```python
from build123d import *

# Parameters (mm, degrees)
F4_DEPTH  = 28.2
F5_R      = 3.9039510248
F6_DEPTH  = 25.8
F7_R      = 5.1903964383
F8_DEPTH  = 37
F10_DEPTH = 2.3
F11_R     = 18.8791722518
F12_DEPTH = 1.5
F13_W     = 2.7272701263
F13_H     = 4.5454557985
F15_R     = 5.8210220824
F16_DEPTH = 19.1
F17_R     = 3.5573808127
F18_DEPTH = 30


with BuildPart() as f1:
    # F0 (on Front) → F1 (revolve)
    with BuildSketch(Plane.XZ):
        with BuildLine():
            Line((-15.875, -15.875), (0, -15.875))
            Line((0, -15.875), (0, 31.75))
            ThreePointArc((0, 31.75), (-11.2253201513, 27.1003201513), (-15.875, 15.875))
            Line((-15.875, 15.875), (-15.875, -15.875))
        make_face()
        with BuildLine():
            Line((0, -31.75), (0, -15.875))
            Line((0, -15.875), (-15.875, -15.875))
            ThreePointArc((-15.875, -15.875), (-11.2253201513, -27.1003201513), (0, -31.75))
        make_face()
    revolve(axis=Axis((0, 0, 0), (0, 0, -1)))

    # F3 (on Front) → F4 (cut)
    with BuildSketch(Plane.XZ):
        with BuildLine():
            add(Edge.make_bspline(
                [(-6.0461172834, 2.4959067814), (-4.028533158, 2.3369491255), (0.1005445797, 2.0116350481), (4.2018322358, 3.6836311663), (6.2991147861, 4.5386427082)],
                knots=[0, 0, 0, 0, 0.4886282733, 1, 1, 1, 1], degree=3))
            add(Edge.make_bspline(
                [(-6.0461172834, 2.4959067814), (-4.1181349295, 1.1140568782), (-0.2700371414, -1.644004442), (5.7694328778, 3.0636466915), (6.1708141175, 4.1813660633), (6.2991147861, 4.5386427082)],
                knots=[0, 0, 0, 0, 0.4058722095, 0.8100883022, 1, 1, 1, 1], degree=3))
        make_face()
    extrude(amount=F4_DEPTH, mode=Mode.SUBTRACT)

    # F5 (on Top) → F6 (join)
    with BuildSketch(Plane.XY):
        with Locations((18.6931826174, 0)):
            Circle(F5_R)
        with Locations((-18.6931826174, 0)):
            Circle(F5_R)
    extrude(amount=-F6_DEPTH)

    # F7 (on Top) → F8 (join)
    with BuildSketch(Plane.XY):
        with Locations((-7.3295454495, 0)):
            Circle(F7_R)
        with Locations((7.3295454495, 0)):
            Circle(F7_R)
    extrude(amount=-F8_DEPTH)

    # F9 (on face) → F10 (join)
    with BuildSketch(Plane(origin=(0, 0, -37), x_dir=(1, 0, 0), z_dir=(0, 0, -1))):
        with BuildLine():
            add(Edge.make_bspline(
                [(-4.4605839066, -4.2878543027), (-3.0017179574, -3.3583444212), (-1.458556714, -0.0316324394), (-2.6367504729, 5.533763177), (-5.0412732751, 9.0001336545), (-10.0021127312, 8.6320191516), (-11.8902083946, 4.7656677042), (-13.3327215963, 0.0556902916), (-10.6600823735, -5.7059711702), (-6.0082775674, -5.2739603612), (-4.4605839066, -4.2878543027)],
                knots=[0, 0, 0, 0, 0.1273841038, 0.2628978132, 0.3751987417, 0.4907069022, 0.6051645787, 0.732271732, 0.8648597083, 1, 1, 1, 1], degree=3))
        make_face()
        with BuildLine():
            add(Edge.make_bspline(
                [(4.4605839066, -4.2878543027), (3.0017179574, -3.3583444212), (1.458556714, -0.0316324394), (2.6367504729, 5.533763177), (5.0412732751, 9.0001336545), (10.0021127312, 8.6320191516), (11.8902083946, 4.7656677042), (13.3327215963, 0.0556902916), (10.6600823735, -5.7059711702), (6.0082775674, -5.2739603612), (4.4605839066, -4.2878543027)],
                knots=[0, 0, 0, 0, 0.1273841038, 0.2628978132, 0.3751987417, 0.4907069022, 0.6051645787, 0.732271732, 0.8648597083, 1, 1, 1, 1], degree=3))
        make_face()
    extrude(amount=F10_DEPTH)

    # F11 (on face) → F12 (join)
    with BuildSketch(Plane(origin=(0, 0, -39.3), x_dir=(1, 0, 0), z_dir=(0, 0, -1))):
        Circle(F11_R)
    extrude(amount=F12_DEPTH)

    # F13 (on Front) → F14 (revolve)
    with BuildSketch(Plane.XZ):
        with Locations((-16.4204556495, 15.1704549789)):
            Rectangle(F13_W, F13_H)
    revolve(axis=Axis((0, 0, 15.9659092315), (0, 0, -1)))

    # F15 (on Front) → F16 (join)
    with BuildSketch(Plane.XZ):
        with Locations((-7.55681796, 16.0795468837)):
            Circle(F15_R)
        with Locations((7.55681796, 16.0795468837)):
            Circle(F15_R)
    extrude(amount=F16_DEPTH)

    # F17 (on Front) → F18 (cut)
    with BuildSketch(Plane.XZ):
        with Locations((-7.55681796, 16.3068193942)):
            Circle(F17_R)
        with Locations((7.55681796, 16.3068193942)):
            Circle(F17_R)
    extrude(amount=F18_DEPTH, mode=Mode.SUBTRACT)


solid = f1.part
```
Geometry: final body of the model. Coordinates: model frame, mm. A direction names the side the tool comes from. Give positions to 0.01 mm unless a question says otherwise; leave off trailing zeros. Write each loop counter-clockwise with the first axis right and the second up, starting at its lowest first coordinate (ties: lowest second). Pieces come first, ordered by that corner, then holes.
1. Draft query along Z for faces 4 (the flat face through (-5.05, -19.1, 13.57)), 5 (the cylindrical face through (-8.02, -9.416, 19.834)), 6 (the flat face through (5.4, 15.1, 17.443)). Return one class per face: released by +Z, released by -Z, zero draft, split by the parting line, or undercut.
2. Section query A-A, the plane y = 12. Return loops of the section in (x, z) (3 decimals), then the cut area to 3 significant figures.
3. Pin query (flat end, axial travel): P1, Ø1.5, axis at x = 7.5, y = -9, coming from the +Z side; P2, Ø2, axis at y = -2.5, z = -11.5, coming from the +X side; P3, Ø1.1, axis at x = 1, y = -17, coming from the +Z side. Return the tip coordinate at first contact, or that it passes through.
4. Reachability of faces 1 (the flat face through (-8, 0, 16)), 2 (the flat face through (0.1, 16.2, 12.898)), 3 (the flat face through (10.1, -19.1, 13.6)) from +Z, -Z, +X, -X, +Y, -Y: full face, straight path, thin tool, end or side. Return the list, or none.
5. Section query B-B, the plane z = -24. Return loops of the section in (x, y).
6. Line query: probe 1 along Z at (x, y) = (-10.5, -13.5); probe 2 along Z at (x, y) = (15.5, -7); probe 3 along X at (y, z) = (-14.5, 18). Output: solid intervals per line, ascending.
Computed:
1. face 4: zero draft
1. face 5: undercut
1. face 6: released by +Z
2. outline: (-14.575, -40.8) - (14.575, -40.8) - (14.575, -39.3) - (-14.575, -39.3) - close; (-13.125, 12.898) - (-10.393, 12.898) - (-10.393, -15.875) arc R10.393 ccw to (10.393, -15.875) - (10.393, 12.898) - (13.125, 12.898) - (13.125, 17.443) - (10.274, 17.443) arc R10.393 ccw to (-10.274, 17.443) - (-13.125, 17.443) - close
2. area: 1,070 mm2
3. P1: stops at z = 27.35
3. P2: stops at x = 22.3
3. P3: stops at z = 17.44
4. face 1: -Y
4. face 2: none
4. face 3: +Z, -Z, +X, -X, -Y
5. outline: circle Ø7.81 at (-18.69, 0); circle Ø27.28 at (0, 0); circle Ø7.81 at (18.69, 0)
6. probe 1: z = -40.8 to -39.3, 11.06 to 14.31, 18.3 to 21.1
6. probe 2: z = -40.8 to -39.3, 12.9 to 17.44
6. probe 3: x = -13.05 to -10.69, -4.43 to 4.43, 10.69 to 13.05
